Could you check a few things on this model? Use its own coordinates, in mm. A direction names the side the tool comes from. Coordinates: 2 decimals unless noted, no trailing zeros. Loops run counter-clockwise (first coordinate to the right, second up) from the corner with the lowest first, then second, coordinate; pieces in that order, holes last. Notation, with made-up numbers: M 85,57 L 104,57 A18 ccw 104,80 Z; hole C 36,88 d4. An arc over 180 degrees is marked long. Return JSON: item names as keys, results as strings. Group by question number.
from build123d import *

# Parameters (mm, degrees)
BOSS_EXTRUDE1_DEPTH = 12
SKETCH3_W           = 20
SKETCH3_H           = 15
BOSS_EXTRUDE2_DEPTH = 1
SKETCH4_W           = 10
SKETCH4_H           = 10
BOSS_EXTRUDE3_DEPTH = 9


with BuildPart() as part:
    # Sketch1 → Boss-Extrude1 (new body)
    with BuildSketch(Plane(origin=(0, 0, 0), x_dir=(1, 0, 0), z_dir=(0, 1, 0))):
        Polygon((3, 2), (18, 2), (18, 13), (3, 13), (3, 11.8), (0, 11.8), (0, 15), (20, 15), (20, 0), (0, 0), (0, 6.7), (3, 6.7), align=None)
    extrude(amount=BOSS_EXTRUDE1_DEPTH)

    # Sketch3 → Boss-Extrude2 (add)
    with BuildSketch(Plane.XZ):
        with Locations((10, -7.5)):
            Rectangle(SKETCH3_W, SKETCH3_H)
    extrude(amount=BOSS_EXTRUDE2_DEPTH)

    # Sketch4 → Boss-Extrude3 (add)
    with BuildSketch(Plane.XZ.offset(1)):
        with Locations((15, -5)):
            Rectangle(SKETCH4_W, SKETCH4_H)
    extrude(amount=BOSS_EXTRUDE3_DEPTH)


solid = part.part
(1) Imagine slicing it at C-C, the plane y = 4.75. Write out the boundary of the cut face in (x, z).
(2) Imagine slicing it at A-A, the plane z = -5. Write out the boundary of the cut face in (x, y).
(3) We'd pull the mould along X, two halves only. Please class faces 1 (the face through (2, 6, -11.8)), 2 (the face through (3, 6, -12)), 3 (the face through (11, 6, -13)), 4 (the face through (20, 1, -6)): +X half, -X half, draft (parallel to the pull), parting line (faces both ways), or undercut.
(4) Imagine slicing it at B-B, the plane x = 4.5. Write out the boundary of the cut face in (y, z), then the cut area to 3 significant figures.
(5) For faces 5 (the face through (10, -5, -5)), 6 (the face through (15, -5, -10)), 7 (the face through (18, 6, -7)), 8 (the face through (1, 6, -6.7)), which set-ups out of +Z, -Z, +X, -X, +Y, -Y let a thin tool reach every point of the face, with its end or its side?
(6) Imagine slicing it at D-D, the plane x = 17.25. Write out the boundary of the cut face in (y, z).
(7) If I drill on L1, parallel to X at y = 8.5, z = -12; L2, parallel to Z at x = 16.5, y = 4.5; L3, parallel to Y at x = 14, z = -5.75, over which ranges is the centre line in solid material (lowest first)? Write a range as [from, to].
(8) Will these pins go through, and if not, where does the flat tip stop? P1, Ø8, axis at x = 12, y = -1.5, coming from the +Z side; P2, Ø7, axis at x = 16.5, y = -5, coming from the -Z side; P3, Ø4.5, axis at y = -4.5, z = -7, coming from the -X side; P4, Ø2, axis at x = 3.5, z = -6, coming from the -Y side.
Checks:
{
 "1": {"outline": "M 0,-15 L 20,-15 L 20,0 L 0,0 L 0,-6.7 L 3,-6.7 L 3,-2 L 18,-2 L 18,-13 L 3,-13 L 3,-11.8 L 0,-11.8 Z"},
 "2": {"outline": "M 0,-1 L 10,-1 L 10,-10 L 20,-10 L 20,12 L 18,12 L 18,0 L 3,0 L 3,12 L 0,12 Z"},
 "3": {"face 1": "draft", "face 2": "undercut", "face 3": "undercut", "face 4": "+X half"},
 "4": {"outline": "M -1,-15 L 12,-15 L 12,-13 L 0,-13 L 0,-2 L 12,-2 L 12,0 L -1,0 Z", "area": "63.0 mm²"},
 "5": {"face 5": "+Z, -Z, -X, -Y", "face 6": "-Z, +X, -X, -Y", "face 7": "+Y", "face 8": "-X, +Y"},
 "6": {"outline": "M -10,-10 L -1,-10 L -1,-15 L 12,-15 L 12,-13 L 0,-13 L 0,-2 L 12,-2 L 12,0 L -10,0 Z"},
 "7": {"L1": "[0, 3], [18, 20]", "L2": "[-15, -13], [-2, 0]", "L3": "[-10, 0]"},
 "8": {"P1": "z = 0", "P2": "z = -10", "P3": "x = 10", "P4": "y = -1"}
}
